Work out the finished part from the listing and answer in its coordinate system (mm). A direction names the side the tool comes from. Coordinates: 2 decimals unless noted, no trailing zeros. Write each loop counter-clockwise with the first axis right and the second up, starting at its lowest first coordinate (ties: lowest second). Pieces come first, ordered by that corner, then holes. Notation, with made-up numbers: (84, 41.5) - (110, 41.5) arc R25 cw to (110, 71.5) - close; hole circle Ø10 at (-14.5, 78). An arc over 180 degrees is marked (long way). Answer as a JSON object with one key per item and string values. Group by question number.
from build123d import *

# Parameters (mm, degrees)
DODANIE_WYCI_GNI_CIE1_DEPTH = 10
SZKIC5_R                    = 1.5
WYTNIJ_WYCI_GNI_CIE2_DEPTH  = 5
SZKIC6_W                    = 7.995239892
SZKIC6_H                    = 7.995239892
WYTNIJ_WYCI_GNI_CIE3_DEPTH  = 6.5


with BuildPart() as part:
    # Szkic1 → Dodanie-wyciągnięcie1 (new body)
    with BuildSketch(Plane(origin=(0, 0, 0), x_dir=(1, 0, 0), z_dir=(0, 1, 0))):
        with BuildLine():
            Line((-25, 0), (25, 0))
            Line((25, 0), (25, 5))
            Line((25, 5), (7.5, 5))
            Line((7.5, 5), (7.5, 11))
            ThreePointArc((7.5, 11), (0, 18.5), (-7.5, 11))
            Line((-7.5, 11), (-7.5, 5))
            Line((-7.5, 5), (-25, 5))
            Line((-25, 5), (-25, 0))
        make_face()
    extrude(amount=DODANIE_WYCI_GNI_CIE1_DEPTH)

    # Szkic5 → Wytnij-wyciągnięcie2 (cut)
    with BuildSketch(Plane(origin=(0, 0, -5), x_dir=(-1, 0, 0), z_dir=(0, 0, -1))):
        with Locations((-21, 5)):
            Circle(SZKIC5_R)
        with Locations((-11.5, 5)):
            Circle(SZKIC5_R)
        with Locations((11.5, 5)):
            Circle(SZKIC5_R)
        with Locations((21, 5)):
            Circle(SZKIC5_R)
    extrude(amount=-WYTNIJ_WYCI_GNI_CIE2_DEPTH, mode=Mode.SUBTRACT)

    # Szkic6 → Wytnij-wyciągnięcie3 (cut)
    with BuildSketch(Plane.XZ):
        with Locations((0, -11)):
            Rectangle(SZKIC6_W, SZKIC6_H)
    extrude(amount=-WYTNIJ_WYCI_GNI_CIE3_DEPTH, mode=Mode.SUBTRACT)


solid = part.part
Q1. For a pull along Y with two mould halves and no side action, classify faces 1 (the face through (0, 0, -5)), 2 (the face through (-19.5, 5.07, -2.54)), 3 (the face through (-7.5, 5, -8)), 4 (the face through (0, 10, -7)) as +Y half, -Y half, draft (parallel to the pull), parting line (faces both ways), or undercut.
Q2. Section B-B on x = -21 is taken. Determine the outline of the cut face in (y, z), plus the area to 3 significant figures.
Q3. A tool of negligible diameter and unlimited length cuts with its end or side. For faces 5 (the face through (0.16, 4.93, -18.5)), 6 (the face through (3.998, 3, -11)), 7 (the face through (13, 5, -3)), 8 (the face through (-16, 5, -5)), 9 (the face through (7.5, 5, -8)), from which of +Z, -Z, +X, -X, +Y, -Y can it reach the whole face along a straight path? Write none if from no direction.
Q4. Consider L1, parallel to Y at x = -11.5, z = -3.65; L2, parallel to X at y = 5.25, z = -10.75; L3, parallel to X at y = 7.75, z = -8.5. Determine where each line is inside the solid, lowest interval first. Write a range as from..to.
Q5. Flat-ended cylindrical pins translate along their axes: pin 1 Ø6 at (x, z) = (8, -5) entering from -Y; pin 2 Ø2.5 at (x, y) = (11.5, 5) entering from -Z; pin 3 Ø3 at (y, z) = (7, -7.5) entering from +X; pin 4 Ø1.5 at (y, z) = (6.5, -7.5) entering from -X. Find the tip coordinate at first contact, or state that the pin passes through.
Q6. Section D-D on y = 8.5 is taken. Determine the outline of the cut face in (x, z), plus the area to 3 significant figures.
Q7. Section A-A on y = 5 is taken. Determine the outline of the cut face in (x, z).
Q8. Section C-C on z = -2.75 is taken. Determine the outline of the cut face in (x, y), plus the area to 3 significant figures.
Numbers:
{
 "1": {"face 1": "-Y half", "face 2": "undercut", "face 3": "draft", "face 4": "+Y half"},
 "2": {"outline": "(0, -5) - (3.5, -5) - (3.5, 0) - (0, 0) - close; (6.5, -5) - (10, -5) - (10, 0) - (6.5, 0) - close", "area": "35.0 mm²"},
 "3": {"face 5": "-Z, +Y, -Y", "face 6": "-Y", "face 7": "+Z, -Z", "face 8": "-Z, -X, +Y, -Y", "face 9": "-Z, +X, +Y, -Y"},
 "4": {"L1": "y = 0..3.5, 6.5..10", "L2": "x = -7.5..-4, 4..7.5", "L3": "x = -7.5..7.5"},
 "5": {"pin 1": "stops at y = 0", "pin 2": "passes through", "pin 3": "stops at x = 7.5", "pin 4": "stops at x = -7.5"},
 "6": {"outline": "(-25, -5) - (-7.5, -5) - (-7.5, -11) arc R7.5 ccw to (7.5, -11) - (7.5, -5) - (25, -5) - (25, 0) - (-25, 0) - close", "area": "428 mm²"},
 "7": {"outline": "(-25, -5) - (-22.5, -5) - (-22.5, 0) - (-25, 0) - close; (-19.5, -5) - (-13, -5) - (-13, 0) - (-19.5, 0) - close; (-10, -5) - (-7.5, -5) - (-7.5, -11) arc R7.5 ccw to (7.5, -11) - (7.5, -5) - (10, -5) - (10, 0) - (-10, 0) - close; (13, -5) - (19.5, -5) - (19.5, 0) - (13, 0) - close; (22.5, -5) - (25, -5) - (25, 0) - (22.5, 0) - close; hole (-4, -15) - (4, -15) - (4, -7) - (-4, -7) - close"},
 "8": {"outline": "(-25, 0) - (25, 0) - (25, 10) - (-25, 10) - close; hole circle Ø3 at (-21, 5); hole circle Ø3 at (-11.5, 5); hole circle Ø3 at (11.5, 5); hole circle Ø3 at (21, 5)", "area": "472 mm²"}
}
